from build123d import *

# Parameters (mm, degrees)
F0_W      = 25.4
F0_H      = 660.4
F1_DEPTH  = 3.175
F2_R      = 9.525
F3_DEPTH  = 25.4
F4_R      = 9.525
F5_DEPTH  = 25.4
F6_R      = 9.525
F7_DEPTH  = 25.4
F8_R      = 9.525
F9_DEPTH  = 25.4
F11_R     = 1.287189
F12_DEPTH = 0.254
F13_R     = 1.283426
F14_DEPTH = 0.254


with BuildPart() as f1:
    # F0 (on Front) → F1 (new body)
    with BuildSketch(Plane.XZ):
        Rectangle(F0_W, F0_H)
    extrude(amount=F1_DEPTH)

    # F2 (on face) → F3 (cut)
    with BuildSketch(Plane.XZ.offset(3.175)):
        with Locations((0, 78.915866)):
            Circle(F2_R)
    extrude(amount=-F3_DEPTH, mode=Mode.SUBTRACT)

    # F4 (on face) → F5 (cut)
    with BuildSketch(Plane.XZ.offset(3.175)):
        with Locations((0, -75.349567)):
            Circle(F4_R)
    extrude(amount=-F5_DEPTH, mode=Mode.SUBTRACT)

    # F6 (on face) → F7 (cut)
    with BuildSketch(Plane.XZ.offset(3.175)):
        with Locations((0, -222.324208)):
            Circle(F6_R)
    extrude(amount=-F7_DEPTH, mode=Mode.SUBTRACT)

    # F8 (on face) → F9 (cut)
    with BuildSketch(Plane(origin=(0, 0, 0), x_dir=(-1, 0, 0), z_dir=(0, 1, 0))):
        with Locations((0, 228.710903)):
            Circle(F8_R)
    extrude(amount=-F9_DEPTH, mode=Mode.SUBTRACT)

    # F11 (on face) → F12 (cut)
    with BuildSketch(Plane.XZ.offset(3.175)):
        with Locations((0, 153.946459)):
            Circle(F11_R)
    extrude(amount=-F12_DEPTH, mode=Mode.SUBTRACT)

    # F13 (on face) → F14 (cut)
    with BuildSketch(Plane.XZ.offset(3.175)):
        with Locations((0, -148.353621)):
            Circle(F13_R)
    extrude(amount=-F14_DEPTH, mode=Mode.SUBTRACT)


solid = f1.part
Source: CAD feature listing. Evaluate the final solid. Frame: model axes, mm. Round coordinates to 2 decimals unless told otherwise and drop trailing zeros. Loops run counter-clockwise (first coordinate to the right, second up) from the corner with the lowest first, then second, coordinate; pieces in that order, holes last. Notation, with made-up numbers: (47, 19) - (72, 19) arc R13 cw to (72, 33) - close; hole circle Ø1 at (53, 36.5). An arc over 180 degrees is marked (long way). Write item = value, one per line. Start each with the question number.
(1) Pull-direction query (X, two-part tool) for faces 1 (the face through (2.06, -1.57, 219.41)), 2 (the face through (-1.24, -1.61, -212.88)), 3 (the face through (0, -3.175, 5)); classes: +X half, -X half, draft (parallel to the pull), parting line (faces both ways), or undercut.
(2) Pin query (flat end, axial travel): pin 1 (1.3 mm diameter, centred on x = -0.5, z = -148.5, fed in from -Y); pin 2 (1 mm diameter, centred on x = -7, z = -205.5, fed in from +Y); pin 3 (11.5 mm diameter, centred on x = 0, z = 228.71, fed in from -Y). Return the tip coordinate at first contact, or that it passes through.
(3) Ray query, line 1 along Z through (x, y) = (0, -2); line 2 along Z through (x, y) = (6.75, -1.5); line 3 along X through (y, z) = (-1.4, 72.5). Return the intervals inside material, ascending. Write a range as from..to.
(4) Section query A-A, the plane y = -0.6. Output: boundary loops of the cut face in (x, z) (3 decimals), plus the area to 3 significant figures.
Conclusion:
q1.face_1 = undercut
q1.face_2 = undercut
q1.face_3 = draft
q2.pin_1 = -2.92
q2.pin_2 = 0
q2.pin_3 = through
q3.line_1 = -330.2..-231.85, -212.8..-84.87, -65.82..69.39, 88.44..219.19, 238.24..330.2
q3.line_2 = -330.2..-229.04, -215.6..-82.07, -68.63..72.2, 85.64..221.99, 235.43..330.2
q3.line_3 = -12.7..-7.04, 7.04..12.7
q4.outline = (-12.7, -330.2) - (12.7, -330.2) - (12.7, 330.2) - (-12.7, 330.2) - close; hole circle Ø19.05 at (0, -222.324); hole circle Ø19.05 at (0, -75.35); hole circle Ø19.05 at (0, 78.916); hole circle Ø19.05 at (0, 228.711)
q4.area = 15,600 mm2
